from build123d import *

# Parameters (mm, degrees)
SKETCH1_W           = 53.34
SKETCH1_H           = 53.34
SKETCH1_R           = 1.9145
SKETCH1_R_2         = 1.75
BOSS_EXTRUDE1_DEPTH = 2.54
FILLET1_R           = 2.54


with BuildPart() as part:
    # Sketch1 → Boss-Extrude1 (new body)
    with BuildSketch(Plane(origin=(0, 0, 0), x_dir=(0, 1, 0), z_dir=(0, 0, 1))):
        Rectangle(SKETCH1_W, SKETCH1_H)
        with Locations((-22.86, -22.86)):
            Circle(SKETCH1_R, mode=Mode.SUBTRACT)
        with Locations((22.86, -22.86)):
            Circle(SKETCH1_R, mode=Mode.SUBTRACT)
        with Locations((22.86, 22.86)):
            Circle(SKETCH1_R, mode=Mode.SUBTRACT)
        with Locations((-22.86, 22.86)):
            Circle(SKETCH1_R, mode=Mode.SUBTRACT)
        with Locations((-15.25, 15.25)):
            Circle(SKETCH1_R_2, mode=Mode.SUBTRACT)
        with Locations((15.25, 15.25)):
            Circle(SKETCH1_R_2, mode=Mode.SUBTRACT)
        with Locations((15.25, -15.25)):
            Circle(SKETCH1_R_2, mode=Mode.SUBTRACT)
        with Locations((-15.25, -15.25)):
            Circle(SKETCH1_R_2, mode=Mode.SUBTRACT)
    extrude(amount=BOSS_EXTRUDE1_DEPTH)

    # Fillet1
    fillet1_edges = [part.edges().sort_by_distance(p)[0] for p in [
        (-26.67, -26.67, 1.27),
        (-26.67, 26.67, 1.27),
        (26.67, 26.67, 1.27),
        (26.67, -26.67, 1.27),
    ]]
    fillet(fillet1_edges, radius=FILLET1_R)


solid = part.part
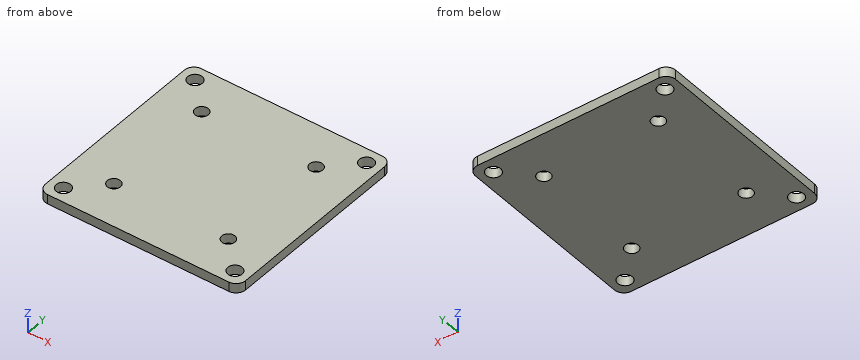
Work out the finished part from the listing and answer in its coordinate system (mm). Give positions to 0.01 mm unless a question says otherwise; leave off trailing zeros. Loops run counter-clockwise (first coordinate to the right, second up) from the corner with the lowest first, then second, coordinate; pieces in that order, holes last. Notation, with made-up numbers: (-30, 82.5) - (-20, 82.5) arc R22 cw to (-20, 111.5) - close; hole circle Ø9 at (70, 86.5). An arc over 180 degrees is marked (long way). Answer in a Markdown table with one row per item. Add a question column.
Q1. Each of these flat-tipped pins is pushed along its axis until it touches: P1, Ø6, axis at x = -22.86, y = -22.86, coming from the -Z side; P2, Ø3, axis at x = -15.25, y = 15.25, coming from the -Z side. Where does it stop, or does it pass through?
Q2. The part is cut by section A-A (y = -22.86). Determine the outline of the cut face in (x, z).
Q3. Consider line 1 along X through (y, z) = (15.25, 2.05); line 2 along Y through (x, z) = (22.86, 1.5). Determine where each line is inside the solid, lowest interval first.
Q4. The part is cut by section B-B (x = -15.25). Determine the outline of the cut face in (y, z).
Q5. The part is cut by section C-C (z = 1.75). State how many separate pieces and enclosed holes the cut face has, and give its area (3 significant figures).
Solution:
| question | item | result |
|---|---|---|
| 1 | P1 | stops at z = 0 |
| 1 | P2 | passes through |
| 2 | outline | (-26.67, 0) - (-24.77, 0) - (-24.77, 2.54) - (-26.67, 2.54) - close; (-20.95, 0) - (20.95, 0) - (20.95, 2.54) - (-20.95, 2.54) - close; (24.77, 0) - (26.67, 0) - (26.67, 2.54) - (24.77, 2.54) - close |
| 3 | line 1 | x = -26.67 to -17, -13.5 to 13.5, 17 to 26.67 |
| 3 | line 2 | y = -26.67 to -24.77, -20.95 to 20.95, 24.77 to 26.67 |
| 4 | outline | (-26.67, 0) - (-17, 0) - (-17, 2.54) - (-26.67, 2.54) - close; (-13.5, 0) - (13.5, 0) - (13.5, 2.54) - (-13.5, 2.54) - close; (17, 0) - (26.67, 0) - (26.67, 2.54) - (17, 2.54) - close |
| 5 | separate pieces | 1 |
| 5 | enclosed holes | 8 |
| 5 | area | 2,760 mm² |
